Build history of the part. All positions in model axes, mm. Face numbers are marked on the shaded views. Coordinates: 2 decimals unless noted, no trailing zeros. Loops run counter-clockwise (first coordinate to the right, second up) from the corner with the lowest first, then second, coordinate; pieces in that order, holes last.
(1) Wall check: L1, parallel to X at y = 0.35, z = 0; L2, parallel to Z at x = 20, y = 0.45; L3, parallel to X at y = 0.3, z = 1. Give the ranges that are in metal, low to high.
(2) Two-plate mould, pull along X, no slides. Class the marked faces 1, 2 and 3: pulls with the +X half, pulls with the -X half, needs draft (parallel to the pull), parting line crosses it, or undercut.
(3) Slice it at B-B (z = 0). Give the cut face in (x, y).
(4) Slice it at A-A (x = 0). Give the cut face in (y, z), and give its area (3 significant figures).
(5) Flat gauge pins, fed straight in: P1, Ø4.5, axis at x = 20, z = 0, coming from the +Y side; P2, Ø2, axis at x = -20, z = 0, coming from the +Y side. Where does each tip first touch, or does it go through?
(6) Slice it at C-C (y = 1.2). Give the cut face in (x, z).
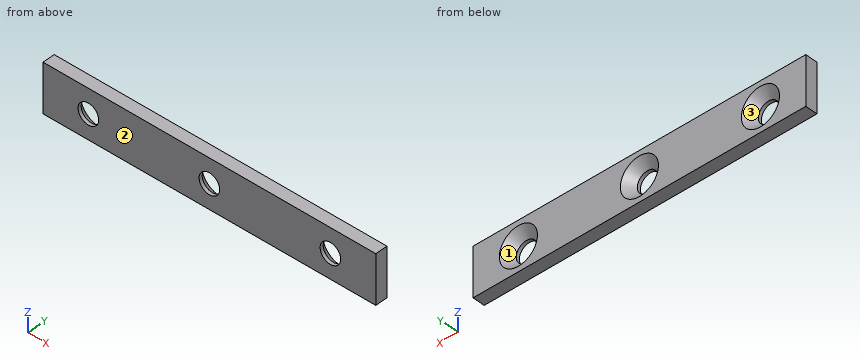
from build123d import *

# Parameters (mm, degrees)
SKETCH1_W           = 55
SKETCH1_H           = 8
BOSS_EXTRUDE1_DEPTH = 2
LPATTERN1_COUNT     = 3
LPATTERN1_PITCH     = 20


with BuildPart() as part:
    # Sketch1 → Boss-Extrude1 (new body)
    with BuildSketch(Plane(origin=(0, 0, 0), x_dir=(1, 0, 0), z_dir=(0, 1, 0))):
        Rectangle(SKETCH1_W, SKETCH1_H)
    extrude(amount=BOSS_EXTRUDE1_DEPTH)

    # Sketch3 → CSK for M3 Countersunk Flat Head1 (revolve, cut)
    with BuildSketch(Plane(origin=(-20, 2, 0), x_dir=(0, 0, 1), z_dir=(1, 0, 0))):
        Polygon((0, 0), (0, 2), (1.7, 2), (1.7, 1.45), (3.15, 0), align=None)
    csk_for_m3_countersunk_flat_head1 = revolve(axis=Axis((-20, 8.35, 0), (0, -1, 0)), mode=Mode.SUBTRACT)

    # LPattern1: CSK for M3 Countersunk Flat Head1 ×3
    with Locations(*[(i * LPATTERN1_PITCH, 0, 0) for i in range(1, LPATTERN1_COUNT)]):
        add(csk_for_m3_countersunk_flat_head1, mode=Mode.SUBTRACT)


solid = part.part
Response values:
1. L1: x = -27.5 to -21.7, -18.3 to -1.7, 1.7 to 18.3, 21.7 to 27.5
1. L2: z = -4 to -1.7, 1.7 to 4
1. L3: x = -27.5 to -21.37, -18.63 to -1.37, 1.37 to 18.63, 21.37 to 27.5
2. face 1: undercut
2. face 2: needs draft
2. face 3: undercut
3. outline: (-27.5, 0) - (-21.7, 0) - (-21.7, 0.55) - (-23.15, 2) - (-27.5, 2) - close; (-18.3, 0) - (-1.7, 0) - (-1.7, 0.55) - (-3.15, 2) - (-16.85, 2) - (-18.3, 0.55) - close; (1.7, 0) - (18.3, 0) - (18.3, 0.55) - (16.85, 2) - (3.15, 2) - (1.7, 0.55) - close; (21.7, 0) - (27.5, 0) - (27.5, 2) - (23.15, 2) - (21.7, 0.55) - close
4. outline: (0, -4) - (2, -4) - (2, -3.15) - (0.55, -1.7) - (0, -1.7) - close; (0, 1.7) - (0.55, 1.7) - (2, 3.15) - (2, 4) - (0, 4) - close
4. area: 7.10 mm2
5. P1: stops at y = 1.1
5. P2: passes through
6. outline: (-27.5, -4) - (27.5, -4) - (27.5, 4) - (-27.5, 4) - close; hole circle Ø4.7 at (-20, 0); hole circle Ø4.7 at (0, 0); hole circle Ø4.7 at (20, 0)
